CAD build for the part. Positions are in the model's coordinates, mm. A direction names the side the tool comes from. Give positions to 0.01 mm unless a question says otherwise; leave off trailing zeros. Loops run counter-clockwise (first coordinate to the right, second up) from the corner with the lowest first, then second, coordinate; pieces in that order, holes last. Notation, with made-up numbers: M 39,17 L 60,17 A20 ccw 60,56 Z; hole C 41,-2.75 d11. An arc over 180 degrees is marked long. Answer as CSV lines item,"result".
Autodesk Inventor part; units mm, degrees
ref_plane "YZ Plane" through (0, 0, 0) normal (1, 0, 0) x (0, 1, 0)
ref_plane "XZ Plane" through (0, 0, 0) normal (0, 1, 0) x (-1, 0, 0)
ref_plane "XY Plane" through (0, 0, 0) normal (0, 0, 1) x (1, 0, 0)
sketch "Sketch1" plane through (0, 0, 0) normal (0, 0, 1) x (1, 0, 0)
  line L0 (-24.5, -14) -> (24.5, -14)
  line L1 (24.5, -14) -> (24.5, 14)
  line L2 (24.5, 14) -> (-24.5, 14)
  line L3 (-24.5, 14) -> (-24.5, -14)
  line L4 (-24.5, -14) -> (24.5, 14) construction
  line L5 (24.5, -14) -> (-24.5, 14) construction
  point P0 (0, 0)
  dimension "d0" = 49
  dimension "d1" = 28
extrude "Extrusion1" add sketch "Sketch1" along normal blind 24.3
sketch "Sketch2" plane through (24.5, -14, 0) normal (1, 0, 0) x (0, 0, -1)
  line L0 (-9, 4.35) -> (-10, 4.35)
  line L1 (-10, 4.35) -> (-10, 10.65)
  line L2 (-10, 10.65) -> (-9, 10.65)
  line L3 (-9, 10.65) -> (-9, 4.35)
  line L4 (-9, 4.35) -> (-10, 10.65) construction
  line L5 (-10, 4.35) -> (-9, 10.65) construction
  line L6 (-9, 17.35) -> (-10, 17.35)
  line L7 (-10, 17.35) -> (-10, 23.65)
  line L8 (-10, 23.65) -> (-9, 23.65)
  line L9 (-9, 23.65) -> (-9, 17.35)
  line L10 (-9, 17.35) -> (-10, 23.65) construction
  line L11 (-10, 17.35) -> (-9, 23.65) construction
  line L12 (-9.5, 7.5) -> (-9.5, 20.5) construction
  line L13 (0, 0) -> (0, 28) construction
  point P0 (0, 14)
  point P1 (-9.5, 14)
  point P2 (0, 14)
  dimension "d4" = 1
  dimension "d5" = 6.3
  dimension "d6" = 6.3
  dimension "d7" = 13
  dimension "d8" = 9
extrude "Extrusion2" add sketch "Sketch2" along normal blind 10
sketch "Sketch3" plane through (-24.5, -14, 0) normal (0, -1, 0) x (1, 0, 0)
  line L0 (19.5, 0) -> (29.5, 0)
  line L1 (29.5, 0) -> (29.5, 1)
  line L2 (29.5, 1) -> (19.5, 1)
  line L3 (19.5, 1) -> (19.5, 0)
  line L4 (0, 0) -> (49, 0)
  point P0 (24.5, 0)
  point P1 (24.5, 0)
  point P2 (24.5, 0)
  point P3 (24.5, 0)
  dimension "d11" = 1
  dimension "d12" = 10
extrude "Extrusion3" add sketch "Sketch3" along normal blind 8.5
sketch "Sketch4" plane through (-24.5, 14, 0) normal (0, 1, 0) x (1, 0, 0)
  line L0 (29.5, -1) -> (29.5, 0)
  line L1 (29.5, 0) -> (19.5, 0)
  line L2 (19.5, 0) -> (19.5, -1)
  line L3 (19.5, -1) -> (29.5, -1)
  line L4 (29.5, -1) -> (29.5, 0)
  line L5 (49, 0) -> (0, 0)
  point P0 (24.5, 0)
  point P1 (24.5, -1)
  point P2 (24.5, 0)
  dimension "d15" = 1
extrude "Extrusion4" add sketch "Sketch4" along normal blind 8.5
sketch "Sketch5" plane through (-24.5, -14, 0) normal (-1, 0, 0) x (0, 0, 1)
  line L0 (12.5, 23.65) -> (13.5, 23.65)
  line L1 (13.5, 23.65) -> (13.5, 17.35)
  line L2 (13.5, 17.35) -> (12.5, 17.35)
  line L3 (12.5, 17.35) -> (12.5, 23.65)
  line L4 (12.5, 23.65) -> (13.5, 17.35) construction
  line L5 (13.5, 23.65) -> (12.5, 17.35) construction
  line L6 (12.5, 4.35) -> (13.5, 4.35)
  line L7 (13.5, 4.35) -> (13.5, 10.65)
  line L8 (13.5, 10.65) -> (12.5, 10.65)
  line L9 (12.5, 10.65) -> (12.5, 4.35)
  line L10 (12.5, 4.35) -> (13.5, 10.65) construction
  line L11 (13.5, 4.35) -> (12.5, 10.65) construction
  line L12 (13, 20.5) -> (13, 7.5) construction
  line L13 (0, 28) -> (0, 0) construction
  point P0 (0, 14)
  point P1 (13, 14)
  point P2 (0, 14)
  dimension "d18" = 1
  dimension "d19" = 6.3
  dimension "d20" = 6.3
  dimension "d21" = 13
  dimension "d22" = 13
extrude "Extrusion5" add sketch "Sketch5" along normal blind 10
sketch "Sketch6" plane through (-24.5, -14, 0) normal (-1, 0, 0) x (0, 0, 1)
  line L0 (23.3, 17.15) -> (24.3, 17.15)
  line L1 (24.3, 17.15) -> (24.3, 10.85)
  line L2 (24.3, 10.85) -> (23.3, 10.85)
  line L3 (23.3, 10.85) -> (23.3, 17.15)
  line L4 (23.3, 17.15) -> (24.3, 10.85) construction
  line L5 (24.3, 17.15) -> (23.3, 10.85) construction
  line L6 (0, 28) -> (0, 0)
  point P0 (0, 14)
  point P1 (23.8, 14)
  point P2 (23.8, 14)
  point P3 (0, 14)
  point P4 (24.3, 28)
  dimension "d25" = 1
  dimension "d26" = 6.3
extrude "Extrusion6" add sketch "Sketch6" along normal blind 10
fillet "Fillet1" radius 1 9 edges at (0, -14, 24.3) (-24.5, -8.575, 24.3) (-24.5, 8.575, 24.3) (-24.5, 14, 12.15) (0, 14, 24.3) (-24.5, -14, 12.15) (24.5, -14, 12.15) (24.5, 0, 24.3) (24.5, 14, 12.15)
fillet "Fillet2" radius 3 8 edges at (5, -14, 0.5) (5, -22.5, 0.5) (-5, -22.5, 0.5) (-5, -14, 0.5) (-5, 14, 0.5) (-5, 22.5, 0.5) (5, 14, 0.5) (5, 22.5, 0.5)
sketch "Sketch7" plane through (0, 0, 0) normal (0, 0, -1) x (-1, 0, 0)
  line L0 (0, 18.5) -> (0, -18.5) construction
  point P0 (0, 0)
  point P1 (0, 0)
  dimension "d31" = 37
hole "Hole1" at (0, 18.5, 0) at (0, -18.5, 0) direction (0, 0, 1) diameter 3.4 depth 8 tip angle 118
properties part number "Netzfilter" material "Aluminum 6061"
Q1. Cut at A-A (x = -28). Write the cut outline in (y, z).
Solution:
outline,"M -9.65,12.5 L -3.35,12.5 L -3.35,13.5 L -9.65,13.5 Z; M -3.15,23.3 L 3.15,23.3 L 3.15,24.3 L -3.15,24.3 Z; M 3.35,12.5 L 9.65,12.5 L 9.65,13.5 L 3.35,13.5 Z"
Q2. Which spindle directions (+Z, -Z, +X, -X, +Y, -Y) get a long thin tool onto all of the face, cutting with end or side? Do faces 1 (the flat face through (0, 16, 1)), 2 (the flat face through (-29, -7, 13.5)), 3 (the flat face through (29, 7, 9)), 4 (the flat face through (-29, -6, 12.5)), 5 (the flat face through (29, -7, 10)). Say none if no direction does.
Solution:
face 1,"+Z, +X, -X, +Y"
face 2,"+Z, -X, +Y, -Y"
face 3,"-Z, +X, +Y, -Y"
face 4,"-Z, -X, +Y, -Y"
face 5,"+Z, +X, +Y, -Y"
Q3. Mould opens along X. For faces 6 (the cylindrical face through (0.65, -16.93, 0.51)), 7 (the cylindrical face through (5.9, 14.86, 0.49)), 8 (the flat face through (0, 14, 11)) say: released by +X, released by -X, zero draft, split by the parting line, or undercut.
Solution:
face 6,"undercut"
face 7,"released by +X"
face 8,"zero draft"
Q4. Wall check: line 1 (Y direction, x = 0, z = 0.35); line 2 (X direction, y = 18.5, z = 0.55); line 3 (X direction, y = 2.5, z = 20.25). Give the ranges that are in metal, low to high. Write a range as [from, to].
Solution:
line 1,"y = [-22.5, -20.2], [-16.8, 16.8], [20.2, 22.5]"
line 2,"x = [-5, -1.7], [1.7, 5]"
line 3,"x = [-24.5, 24.5]"
Q5. Pin check, flat tips, straight feed: P1, Ø5, axis at x = 28.5, y = 7, coming from the +Z side; P2, Ø3, axis at x = -15, z = 18, coming from the +Y side; P3, Ø3, axis at x = 12.5, y = -15, coming from the -Z side; P4, Ø4, axis at y = 1.5, z = 19.5, coming from the -X side. Stop position of each tip, or through.
Solution:
P1,"stops at z = 10"
P2,"stops at y = 14"
P3,"stops at z = 0"
P4,"stops at x = -24.5"
Q6. Cut at C-C (z = 22). Write the cut outline in (x, y).
Solution:
outline,"M -24.5,-13 A1 ccw -23.5,-14 L 23.5,-14 A1 ccw 24.5,-13 L 24.5,13 A1 ccw 23.5,14 L -23.5,14 A1 ccw -24.5,13 Z"
Q7. Cut at D-D (x = 27.5). Write the cut outline in (y, z).
Solution:
outline,"M -9.65,9 L -3.35,9 L -3.35,10 L -9.65,10 Z; M 3.35,9 L 9.65,9 L 9.65,10 L 3.35,10 Z"
Q8. Cut at B-B (y = 18.5). Write the cut outline in (x, z).
Solution:
outline,"M -5,0 L -1.7,0 L -1.7,1 L -5,1 Z; M 1.7,0 L 5,0 L 5,1 L 1.7,1 Z"
